Verification items for the finished model (mm, model axes). A direction names the side the tool comes from. Coordinates: 2 decimals unless noted, no trailing zeros. Write each loop counter-clockwise with the first axis right and the second up, starting at its lowest first coordinate (ties: lowest second). Pieces come first, ordered by that corner, then holes. Notation, with made-up numbers: (6, 41.5) -> (25, 41.5) arc R18 cw to (25, 56.5) -> close; hole circle Ø5 at (52.5, -36.75). An arc over 180 degrees is marked (long way). Write each question's results on one line, items separated by ' | '. Start each with the question number.
from build123d import *

# Parameters (mm, degrees)
SKETCH1_R           = 30
SKETCH1_R_2         = 15.5
BOSS_EXTRUDE1_DEPTH = 10
BOSS_EXTRUDE2_DEPTH = 10
SKETCH3_W           = 15
SKETCH3_H           = 2
SKETCH4_W           = 1.6
SKETCH4_H           = 1.9
FILLET1_R           = 5


with BuildPart() as part:
    # Sketch1 → Boss-Extrude1 (new, symmetric)
    with BuildSketch(Plane.XY):
        Circle(SKETCH1_R)
        Circle(SKETCH1_R_2, mode=Mode.SUBTRACT)
    extrude(amount=BOSS_EXTRUDE1_DEPTH, both=True)

    # Sketch2 → Boss-Extrude2 (add, symmetric)
    with BuildSketch(Plane.XY):
        Polygon((-8, 100), (8, 100), (8, 28.91366459), (0, 30), (-8, 28.91366459), align=None)
    boss_extrude2 = extrude(amount=BOSS_EXTRUDE2_DEPTH, both=True)

    # Mirror1: Boss-Extrude2 across plane
    add(boss_extrude2.mirror(Plane.ZX))

    # Sketch3 → Cut-Revolve1 (revolve, cut)
    with BuildSketch(Plane(origin=(0, 0, 0), x_dir=(0, 0, -1), z_dir=(1, 0, 0)), mode=Mode.PRIVATE) as cut_revolve1_sk:
        with Locations((-2.5, 16.5)):
            Rectangle(SKETCH3_W, SKETCH3_H)
    revolve(cut_revolve1_sk.sketch.rotate(Axis((0, 0, 0), (0, 0, -1)), 90), axis=Axis((0, 0, 0), (0, 0, -1)), mode=Mode.SUBTRACT)

    # Sketch4 → Cut-Revolve2 (revolve, cut)
    with BuildSketch(Plane(origin=(0, 0, 0), x_dir=(0, 0, -1), z_dir=(1, 0, 0)), mode=Mode.PRIVATE) as cut_revolve2_sk:
        with Locations((-5.7, 17.95)):
            Rectangle(SKETCH4_W, SKETCH4_H)
    revolve(cut_revolve2_sk.sketch.rotate(Axis((0, 0, 0), (0, 0, -1)), 90), axis=Axis((0, 0, 0), (0, 0, -1)), mode=Mode.SUBTRACT)

    # Fillet1
    fillet1_edges = [part.edges().sort_by_distance(p)[0] for p in [
        (8, 28.91366459, 0),
        (-8, 28.91366459, 0),
        (8, -28.91366459, 0),
        (-8, -28.91366459, 0),
    ]]
    fillet(fillet1_edges, radius=FILLET1_R)


solid = part.part
1. Mould release check, pull along X, two halves, no side actions. Record for faces 1 (the cylindrical face through (8.836, -29.728, -0.14)), 2 (the cylindrical face through (-8.836, -29.728, 0.14)), 3 (the cylindrical face through (-3.794, 17.084, -0.119)): +X half, -X half, draft (parallel to the pull), parting line (faces both ways), or undercut.
2. Sectioned sample at C-C on x = 0. Record the cut outline in (y, z), plus the area to 3 significant figures.
3. Depth check by flat-ended pin: pin 1 Ø6 at (y, z) = (61, -4.5) entering from -X; pin 2 Ø2 at (x, z) = (23, -6.5) entering from -Y; pin 3 Ø4 at (x, z) = (23, -4.5) entering from +Y. Enter the tip coordinate at first touch or a pass-through.
4. Sectioned sample at B-B on z = 2.25. Record the cut outline in (x, y), plus the area to 3 significant figures.
5. Material ranges on probe 1 along Y at (x, z) = (0, 8.95); probe 2 along Y at (x, z) = (0, -8.45); probe 3 along X at (y, z) = (1, -6), recorded low to high. Write a range as from..to.
6. Tool access check on faces 4 (the flat face through (8, 67, 0)), 5 (the flat face through (7, 14, -5)), 6 (the flat face through (8, -67, 0)), 7 (the flat face through (-8, 66, 0)). Record the directions out of +Z, -Z, +X, -X, +Y, -Y that give a thin tool (end or side, any length) a straight path to the whole face; none if there is none.
7. Sectioned sample at A-A on y = 0. Record the cut outline in (x, z).
8. Sectioned sample at D-D on y = 42. Record the cut outline in (x, z).
Computed values:
1) face 1: +X half | face 2: -X half | face 3: undercut
2) outline: (-100, -10) -> (-15.5, -10) -> (-15.5, -5) -> (-17.5, -5) -> (-17.5, 4.9) -> (-18.9, 4.9) -> (-18.9, 6.5) -> (-17.5, 6.5) -> (-17.5, 10) -> (-100, 10) -> close; (15.5, -10) -> (100, -10) -> (100, 10) -> (17.5, 10) -> (17.5, 6.5) -> (18.9, 6.5) -> (18.9, 4.9) -> (17.5, 4.9) -> (17.5, -5) -> (15.5, -5) -> close | area: 3,320 mm^2
3) pin 1: stops at x = -8 | pin 2: stops at y = -20.4 | pin 3: stops at y = 21.42
4) outline: (-11.14, -27.85) arc R5 cw to (-8, -32.5) -> (-8, -100) -> (8, -100) -> (8, -32.5) arc R5 cw to (11.14, -27.85) arc R30 ccw to (11.14, 27.85) arc R5 cw to (8, 32.5) -> (8, 100) -> (-8, 100) -> (-8, 32.5) arc R5 cw to (-11.14, 27.85) arc R30 ccw to start; hole circle Ø35 at (0, 0) | area: 4,130 mm^2
5) probe 1: y = -100..-17.5, 17.5..100 | probe 2: y = -100..-15.5, 15.5..100 | probe 3: x = -29.98..-15.47, 15.47..29.98
6) face 4: +Z, -Z, +X, +Y | face 5: +Z | face 6: +Z, -Z, +X, -Y | face 7: +Z, -Z, -X, +Y
7) outline: (-30, -10) -> (-15.5, -10) -> (-15.5, -5) -> (-17.5, -5) -> (-17.5, 4.9) -> (-18.9, 4.9) -> (-18.9, 6.5) -> (-17.5, 6.5) -> (-17.5, 10) -> (-30, 10) -> close; (15.5, -10) -> (30, -10) -> (30, 10) -> (17.5, 10) -> (17.5, 6.5) -> (18.9, 6.5) -> (18.9, 4.9) -> (17.5, 4.9) -> (17.5, -5) -> (15.5, -5) -> close
8) outline: (-8, -10) -> (8, -10) -> (8, 10) -> (-8, 10) -> close
